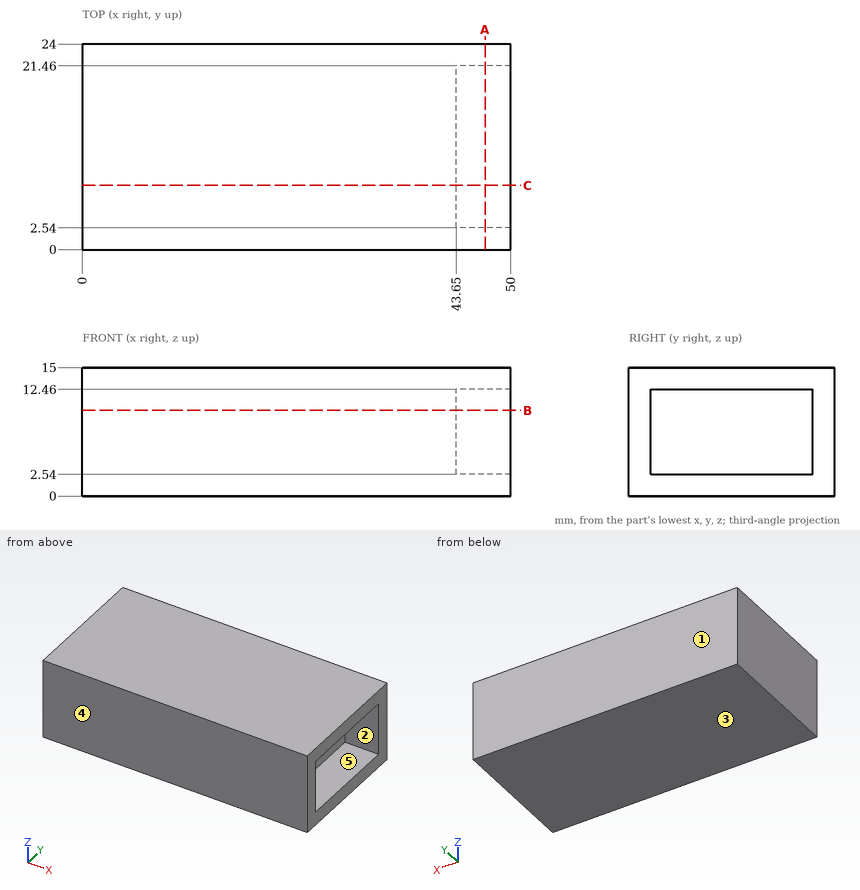
Design review of the part shown in the three views and the two pictorial views. Dimensions are in mm from the part's minimum x, y and z. A direction names the side the tool comes from. Coordinates: 2 decimals unless noted, no trailing zeros. Loops run counter-clockwise (first coordinate to the right, second up) from the corner with the lowest first, then second, coordinate; pieces in that order, holes last. Notation, with made-up numbers: M 40,-15.75 L 93,-15.75 A26 cw 93,1.25 Z; hole C -25,29 d6. An arc over 180 degrees is marked long. Put each result on its own line as item: value. Start each with the question number.
Q1. Wall thickness on line 1 (Z direction, x = 45, y = 5.5); line 2 (Y direction, x = 46, z = 9.5); line 3 (X direction, y = 11, z = 7.75): over which ranges is each line inside the solid? List them lowest first.
Q2. Add section A-A (x = 47). Write out the cut boundary in (y, z).
Q3. Add section C-C (y = 7.5). Write out the cut boundary in (x, z).
Q4. Add section B-B (z = 10). Write out the cut boundary in (x, y).
Q5. Clearance check with a flat-ended pin moving along its axis: pin 1 (3 mm diameter, centred on y = 16.5, z = 8.5, fed in from +X). State where the tip first meets the part, or that it passes through.
Q6. The part is to be moulded in two halves that separate along Y. For the marked faces 1, 2 and 3, say which applies: +Y half, -Y half, draft (parallel to the pull), parting line (faces both ways), or undercut.
Q7. For the marked faces 4 and 5, list the 3-axis set-ups (+Z, -Z, +X, -X, +Y, -Y) from which the entire face can be reached by the end or side of a thin tool; tool diameter is ignored.
Answers:
1. line 1: z = 0 to 2.54, 12.46 to 15
1. line 2: y = 0 to 2.54, 21.46 to 24
1. line 3: x = 0 to 43.65
2. outline: M 0,0 L 24,0 L 24,15 L 0,15 Z; hole M 2.54,2.54 L 21.46,2.54 L 21.46,12.46 L 2.54,12.46 Z
3. outline: M 0,0 L 50,0 L 50,2.54 L 43.65,2.54 L 43.65,12.46 L 50,12.46 L 50,15 L 0,15 Z
4. outline: M 0,0 L 50,0 L 50,2.54 L 43.65,2.54 L 43.65,21.46 L 50,21.46 L 50,24 L 0,24 Z
5. pin 1: stops at x = 43.65
6. face 1: +Y half
6. face 2: undercut
6. face 3: draft
7. face 4: +Z, -Z, +X, -X, -Y
7. face 5: +X
